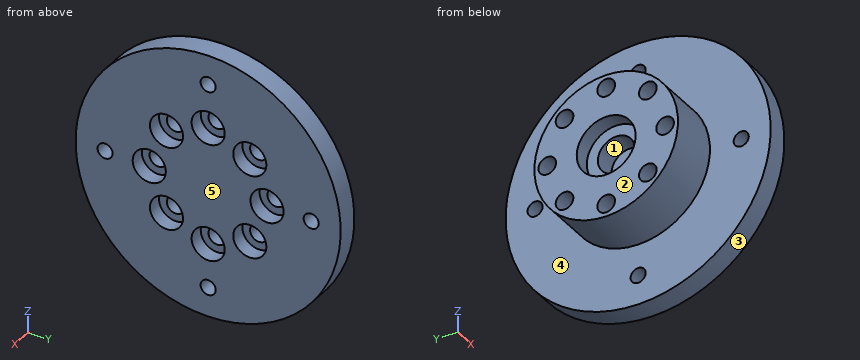
from build123d import *

# Parameters (mm, degrees)
SKETCH1_R                                       = 9.75
BOSS_EXTRUDE1_DEPTH                             = 10
SKETCH6_R                                       = 18
BOSS_EXTRUDE2_DEPTH                             = 3
CBORE_FOR_M2_SOCKET_HEAD_CAP_SCREW5_D           = 2.4
CBORE_FOR_M2_SOCKET_HEAD_CAP_SCREW5_CBORE_D     = 4.5
CBORE_FOR_M2_SOCKET_HEAD_CAP_SCREW5_CBORE_DEPTH = 2
SKETCH14_R                                      = 4
CUT_EXTRUDE1_DEPTH                              = 2.2
M2_5_TAPPED_HOLE1_D                             = 2.05
SKETCH16_R                                      = 2.5
CUT_EXTRUDE2_DEPTH                              = 3


with BuildPart() as part:
    # Sketch1 → Boss-Extrude1 (new body)
    with BuildSketch(Plane(origin=(0, 0, 0), x_dir=(0, 0, -1), z_dir=(1, 0, 0))):
        Circle(SKETCH1_R)
    extrude(amount=BOSS_EXTRUDE1_DEPTH)

    # Sketch6 → Boss-Extrude2 (add)
    with BuildSketch(Plane(origin=(7, 0, 0), x_dir=(0, 0, -1), z_dir=(1, 0, 0))):
        Circle(SKETCH6_R)
    extrude(amount=BOSS_EXTRUDE2_DEPTH)

    # CBORE for M2 Socket Head Cap Screw5 (through all)
    with Locations(Plane(origin=(10, 8, 0), x_dir=(0, 0, 1), z_dir=(1, 0, 0))):
        with Locations((0, 0), (-5.656854249, 2.343145751), (-8, 8), (-5.656854249, 13.656854249), (0, 16), (5.656854249, 13.656854249), (8, 8), (5.656854249, 2.343145751)):
            CounterBoreHole(CBORE_FOR_M2_SOCKET_HEAD_CAP_SCREW5_D / 2, CBORE_FOR_M2_SOCKET_HEAD_CAP_SCREW5_CBORE_D / 2, CBORE_FOR_M2_SOCKET_HEAD_CAP_SCREW5_CBORE_DEPTH)

    # Sketch14 → Cut-Extrude1 (cut)
    with BuildSketch(Plane.ZY):
        Circle(SKETCH14_R)
    extrude(amount=-CUT_EXTRUDE1_DEPTH, mode=Mode.SUBTRACT)

    # M2.5 Tapped Hole1 (through all)
    with Locations(Plane(origin=(10, 14, 0), x_dir=(0, 0, 1), z_dir=(1, 0, 0))):
        with Locations((0, 0), (-14, 14), (0, 28), (14, 14)):
            Hole(M2_5_TAPPED_HOLE1_D / 2)

    # Sketch16 → Cut-Extrude2 (cut)
    with BuildSketch(Plane(origin=(2.2, 0, 0), x_dir=(0, 0, -1), z_dir=(1, 0, 0))):
        Circle(SKETCH16_R)
    extrude(amount=CUT_EXTRUDE2_DEPTH, mode=Mode.SUBTRACT)


solid = part.part
Here's how the part is built. I have some questions about the finished solid (model axes, mm). Face numbers are marked on the shaded views. A direction names the side the tool comes from. Round coordinates to 2 decimals unless told otherwise and drop trailing zeros. Loops run counter-clockwise (first coordinate to the right, second up) from the corner with the lowest first, then second, coordinate; pieces in that order, holes last.
1. We'd pull the mould along Z, two halves only. Please class the marked faces 1, 2 and 3: +Z half, -Z half, draft (parallel to the pull), parting line (faces both ways), or undercut.
Answer list:
face 1: undercut
face 2: draft
face 3: parting line
2. If we section it at A-A on z = -14: Write out the boundary of the cut face in (x, y) (3 decimals).
Answer list:
outline: (7, -11.314) - (10, -11.314) - (10, -1.025) - (7, -1.025) - close; (7, 1.025) - (10, 1.025) - (10, 11.314) - (7, 11.314) - close
3. If I drill on line 1 along Y through (x, z) = (4.75, 0); line 2 along Y through (x, z) = (8.1, 0) (3 decimals); line 3 along Z through (x, y) = (2.25, -0.5), over which ranges is the centre line in solid material (lowest first)?
Answer list:
line 1: y = -9.75 to -9.2, -6.8 to -2.5, 2.5 to 6.8, 9.2 to 9.75
line 2: y = -18 to -15.025, -12.975 to -10.25, -5.75 to 5.75, 10.25 to 12.975, 15.025 to 18
line 3: z = -9.74 to -9.09, -6.91 to -2.45, 2.45 to 6.91, 9.09 to 9.74
4. If we section it at B-B on x = 7.5: Count the separate pieces of the cut face and the enclosed holes in it, plus the area to 3 significant figures.
Answer list:
separate pieces: 1
enclosed holes: 12
area: 968 mm2
5. Which directions (+Z, -Z, +X, -X, +Y, -Y) give clear straight access to the entire face, cutting with the end or side of a thin tool? Please do the marked faces 4 and 5.
Answer list:
face 4: -X
face 5: +Z, -Z, +X, +Y, -Y
6. For P1, Ø4, axis at x = 4.5, y = 1, coming from the -Z side; P2, Ø2.5, axis at y = 2, z = -1.5, coming from the -X side; P3, Ø4, axis at x = 5.5, y = 3, coming from the +Z side, each with a flat end and sliding along its axis, tell me the tip position at first contact or that it passes through.
Answer list:
P1: stops at z = -9.75
P2: stops at x = 2.2
P3: stops at z = 17.92
